For this review, take the finished solid that the model builds, in its own axes (mm). Round coordinates to 2 decimals unless told otherwise and drop trailing zeros. Loops run counter-clockwise (first coordinate to the right, second up) from the corner with the lowest first, then second, coordinate; pieces in that order, holes last.
1) Take a section at B-B (y = 2.6). State the section outline as (x, z) points.
2) Take a section at C-C (z = 58.5). State the section outline as (x, y) points, then the cut area to 3 significant figures.
3) Take a section at A-A (x = 3). State the section outline as (y, z) points.
4) Wall thickness on L1, parallel to X at y = 0.6, z = 58.5; L2, parallel to Z at x = 91.4, y = 1.3; L3, parallel to Y at x = 6, z = 59: over which ranges is each line inside the solid? List them lowest first.
5) Insertion check: pin 1 (1 mm diameter, centred on y = 3, z = 44, fed in from +X); pin 2 (0.6 mm diameter, centred on y = 2, z = 23.5, fed in from +X); pin 3 (5 mm diameter, centred on x = 50, z = 37, fed in from +Y). Each pin has a flat end and moves straight along its axis. Give the tip position at first contact, or say it passes through.
6) Take a section at D-D (x = 91.4). State the section outline as (y, z) points, then the cut area to 3 significant figures.
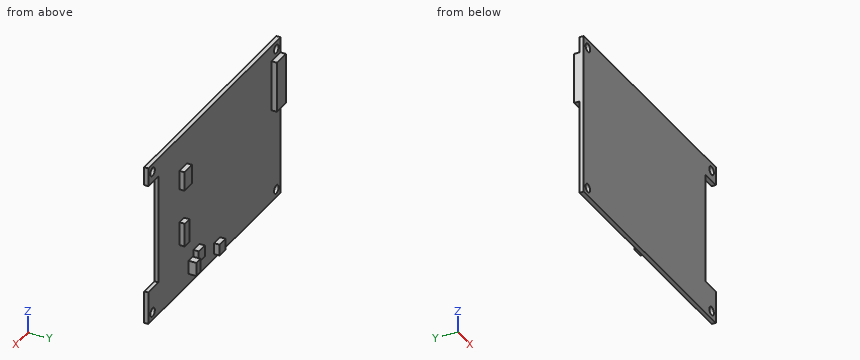
```python
from build123d import *

# Parameters (mm, degrees)
SKETCH_1_R      = 1.6
EXTRUDE_1_DEPTH = 1.6
SKETCH_2_W      = 6.4
SKETCH_2_H      = 19.4
SKETCH_2_W_2    = 5.4
SKETCH_2_H_2    = 7.3
SKETCH_2_W_3    = 3.3
SKETCH_2_H_3    = 9
SKETCH_2_W_4    = 4.3
SKETCH_2_H_4    = 4.3
EXTRUDE_2_DEPTH = 2
SKETCH_3_W      = 3
SKETCH_3_H      = 5.2
EXTRUDE_3_DEPTH = 3


with BuildPart() as part:
    # 草图1 → 凸台-拉伸1 (new body)
    with BuildSketch(Plane(origin=(0, 0, 0), x_dir=(1, 0, 0), z_dir=(0, 1, 0))):
        Polygon((94.4, 0), (0, 0), (0, -61.5), (94.4, -61.5), (94.4, -54.45), (87.2, -54.45), (87.2, -12.45), (94.4, -12.45), align=None)
        with Locations(Location((3, -58.5, 0), (0, 0, 270))):
            Circle(SKETCH_1_R, mode=Mode.SUBTRACT)
        with Locations(Location((91.4, -58.5, 0), (0, 0, 270))):
            Circle(SKETCH_1_R, mode=Mode.SUBTRACT)
        with Locations(Location((3, -3, 0), (0, 0, 270))):
            Circle(SKETCH_1_R, mode=Mode.SUBTRACT)
        with Locations(Location((91.4, -3, 0), (0, 0, 270))):
            Circle(SKETCH_1_R, mode=Mode.SUBTRACT)
    extrude(amount=EXTRUDE_1_DEPTH)

    # 草图2 → 凸台-拉伸2 (add)
    with BuildSketch(Plane(origin=(0, 1.6, 0), x_dir=(1, 0, 0), z_dir=(0, 1, 0))):
        with Locations((3.2, -45.8)):
            Rectangle(SKETCH_2_W, SKETCH_2_H)
        with Locations((69.6, -44.75)):
            Rectangle(SKETCH_2_W_2, SKETCH_2_H_2)
        with Locations((70.55, -23.5)):
            Rectangle(SKETCH_2_W_3, SKETCH_2_H_3)
        with Locations((45.25, -3.95)):
            Rectangle(SKETCH_2_W_4, SKETCH_2_H_4)
        with Locations((60.05, -9.45)):
            Rectangle(SKETCH_2_W_4, SKETCH_2_H_4)
    extrude(amount=EXTRUDE_2_DEPTH)

    # 草图3 → 凸台-拉伸3 (add)
    with BuildSketch(Plane(origin=(0, 1.6, 0), x_dir=(1, 0, 0), z_dir=(0, 1, 0))):
        with Locations((64.3, -6.7)):
            Rectangle(SKETCH_3_W, SKETCH_3_H)
    extrude(amount=EXTRUDE_3_DEPTH)


solid = part.part
```
Response:
1. outline: (0, 36.1) - (6.4, 36.1) - (6.4, 55.5) - (0, 55.5) - close; (43.1, 1.8) - (47.4, 1.8) - (47.4, 6.1) - (43.1, 6.1) - close; (57.9, 7.3) - (62.2, 7.3) - (62.2, 11.6) - (57.9, 11.6) - close; (62.8, 4.1) - (65.8, 4.1) - (65.8, 9.3) - (62.8, 9.3) - close; (66.9, 41.1) - (72.3, 41.1) - (72.3, 48.4) - (66.9, 48.4) - close; (68.9, 19) - (72.2, 19) - (72.2, 28) - (68.9, 28) - close
2. outline: (0, 0) - (1.4, 0) - (1.4, 1.6) - (0, 1.6) - close; (4.6, 0) - (89.8, 0) - (89.8, 1.6) - (4.6, 1.6) - close; (93, 0) - (94.4, 0) - (94.4, 1.6) - (93, 1.6) - close
2. area: 141 mm2
3. outline: (0, 0) - (1.6, 0) - (1.6, 1.4) - (0, 1.4) - close; (0, 4.6) - (1.6, 4.6) - (1.6, 36.1) - (3.6, 36.1) - (3.6, 55.5) - (1.6, 55.5) - (1.6, 56.9) - (0, 56.9) - close; (0, 60.1) - (1.6, 60.1) - (1.6, 61.5) - (0, 61.5) - close
4. L1: x = 0 to 1.4, 4.6 to 89.8, 93 to 94.4
4. L2: z = 0 to 1.4, 4.6 to 12.45, 54.45 to 56.9, 60.1 to 61.5
4. L3: y = 0 to 1.6
5. pin 1: stops at x = 72.3
5. pin 2: stops at x = 72.2
5. pin 3: stops at y = 1.6
6. outline: (0, 0) - (1.6, 0) - (1.6, 1.4) - (0, 1.4) - close; (0, 4.6) - (1.6, 4.6) - (1.6, 12.45) - (0, 12.45) - close; (0, 54.45) - (1.6, 54.45) - (1.6, 56.9) - (0, 56.9) - close; (0, 60.1) - (1.6, 60.1) - (1.6, 61.5) - (0, 61.5) - close
6. area: 21.0 mm2
